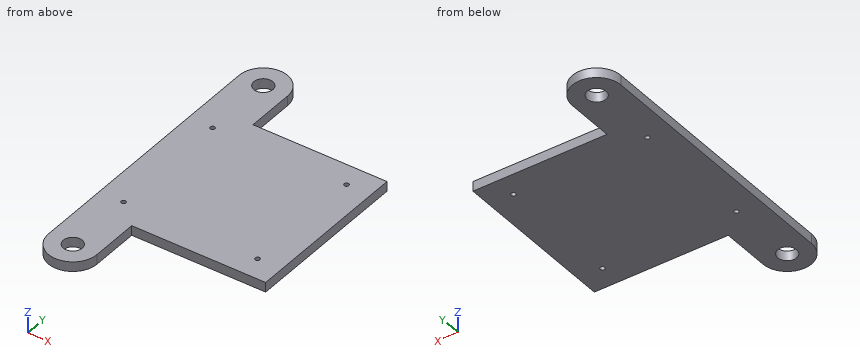
```python
from build123d import *

# Parameters (mm, degrees)
SKETCH1_W                      = 27.56
SKETCH1_H                      = 34.956966618
BOSS_EXTRUDE1_DEPTH            = 2
TAP_DRILL_FOR_M1_2X0_25_TAP2_D = 0.95
M3_5_CLEARANCE_HOLE1_D         = 3.9


with BuildPart() as part:
    # Sketch1 → Boss-Extrude1 (new body)
    with BuildSketch(Plane.XY):
        with Locations((5, 0)):
            Rectangle(SKETCH1_W, SKETCH1_H)
        Polygon((-18.78, -10), (-18.78, -17.478483309), (-8.78, -17.478483309), (-8.78, 17.478483309), (-18.78, 17.478483309), (-18.78, 10), align=None)
        with BuildLine():
            Line((-18.78, 17.478483309), (-8.78, 17.478483309))
            Line((-8.78, 17.478483309), (-8.78, 27.45))
            ThreePointArc((-8.78, 27.45), (-13.78, 32.45), (-18.78, 27.45))
            Line((-18.78, 27.45), (-18.78, 17.478483309))
        make_face()
        with BuildLine():
            Line((-8.78, -17.478483309), (-18.78, -17.478483309))
            Line((-18.78, -17.478483309), (-18.78, -27.45))
            ThreePointArc((-18.78, -27.45), (-13.78, -32.45), (-8.78, -27.45))
            Line((-8.78, -27.45), (-8.78, -17.478483309))
        make_face()
    extrude(amount=BOSS_EXTRUDE1_DEPTH)

    # Tap Drill for M1.2x0.25 Tap2 (through all)
    with Locations(Plane.XY.offset(2)):
        with Locations((-13.78, -12.825), (-13.78, 12.825), (13.78, 12.825), (13.78, -12.825)):
            Hole(TAP_DRILL_FOR_M1_2X0_25_TAP2_D / 2)

    # M3.5 Clearance Hole1 (through all)
    with Locations(Plane.XY.offset(2)):
        with Locations((-13.78, -27.45), (-13.78, 27.45)):
            Hole(M3_5_CLEARANCE_HOLE1_D / 2)


solid = part.part
```
CAD build for the part. Positions are in the model's coordinates, mm. Round coordinates to 2 decimals unless told otherwise and drop trailing zeros. Order: outer loops, then holes, each group sorted by start corner. A loop starts at its lowest first (then second) coordinate and runs counter-clockwise, first axis right, second up.
Q1. Wall check: L1, parallel to Y at x = -13.78, z = 0.4; L2, parallel to Y at x = 13.78, z = 0.95; L3, parallel to Y at x = -12, z = 0.5. Give the ranges that are in metal, low to high.
Q2. Slice it at A-A (z = 0.4). Write the cut outline in (x, y) (3 decimals), and give its area (3 significant figures).
Q3. Drop flat-ended pins along their axis: pin 1 (1 mm diameter, centred on x = -1.5, z = 1.5, fed in from -Y); pin 2 (0.6 mm diameter, centred on y = -23.5, z = 1, fed in from +X). Give the stop position or say it passes through.
Q4. Slice it at B-B (x = 15). Write the cut outline in (y, z), and give its area (3 significant figures).
Results below:
1. L1: y = -32.45 to -29.4, -25.5 to -13.3, -12.35 to 12.35, 13.3 to 25.5, 29.4 to 32.45
1. L2: y = -17.48 to -13.3, -12.35 to 12.35, 13.3 to 17.48
1. L3: y = -32.12 to -28.25, -26.65 to 26.65, 28.25 to 32.12
2. outline: (-18.78, -27.45) arc R5 ccw to (-8.78, -27.45) - (-8.78, -17.478) - (18.78, -17.478) - (18.78, 17.478) - (-8.78, 17.478) - (-8.78, 27.45) arc R5 ccw to (-18.78, 27.45) - close; hole circle Ø3.9 at (-13.78, -27.45); hole circle Ø3.9 at (-13.78, 27.45); hole circle Ø0.95 at (-13.78, -12.825); hole circle Ø0.95 at (-13.78, 12.825); hole circle Ø0.95 at (13.78, -12.825); hole circle Ø0.95 at (13.78, 12.825)
2. area: 1,560 mm2
3. pin 1: stops at y = -17.48
3. pin 2: stops at x = -8.78
4. outline: (-17.48, 0) - (17.48, 0) - (17.48, 2) - (-17.48, 2) - close
4. area: 69.9 mm2
